For this review, take the finished solid that the model builds, in its own axes (mm). Face numbers are marked on the shaded views. A direction names the side the tool comes from. Round coordinates to 2 decimals unless told otherwise and drop trailing zeros. Order: outer loops, then holes, each group sorted by start corner. A loop starts at its lowest first (then second) coordinate and runs counter-clockwise, first axis right, second up. Notation, with made-up numbers: (42.5, 68) -> (85.5, 68) arc R26 cw to (85.5, 93) -> close; hole circle Ø10 at (42.25, 53). An arc over 180 degrees is marked (long way). Use a Markdown table: item, result. Add a question column.
1) Consider section A-A (z = -10.5). State the section outline as (x, y) points.
2) Draft analysis for pull direction X (two halves, no side actions). For the marked faces 6, 7 and 8, state which applies: pulls with the +X half, pulls with the -X half, needs draft (parallel to the pull), parting line crosses it, or undercut.
3) Consider section C-C (y = 12.5). State the section outline as (x, z) points, plus the area to 3 significant figures.
4) Clearance check with flat-ended pins moving along their axes: P1, Ø2, axis at y = 12.5, z = -7.5, coming from the -X side; P2, Ø6, axis at x = -32.5, z = 9.5, coming from the -Y side; P3, Ø2, axis at y = 2, z = -11, coming from the +X side; P4, Ø5, axis at x = -27, y = 9.5, coming from the +Z side. State where each tip first meets the part, or that it passes through.
5) Wall thickness on line 1 along X through (y, z) = (2.15, -10.5); line 2 along Y through (x, z) = (-28, -9); line 3 along Z through (x, y) = (-24, 12.5): over which ranges is each line inside the solid? List them lowest first. Write a range as [from, to].
6) Machinability: for the marked faces 1, 2, 3, 4 and 5, which of the approach directions +Z, -Z, +X, -X, +Y, -Y give a long, thin tool a straight path to every point of the face, cutting with its end or side? Answer none if there is none.
```python
from build123d import *

# Parameters (mm, degrees)
SKETCH1_W           = 15
SKETCH1_H           = 26
BOSS_EXTRUDE1_DEPTH = 3
CUT_EXTRUDE1_REACH  = 39.924
SKETCH2_R           = 1
SKETCH3_W           = 5
SKETCH3_H           = 10
BOSS_EXTRUDE2_DEPTH = 16
CUT_EXTRUDE2_REACH  = 29.477
SKETCH4_R           = 3
CUT_EXTRUDE3_REACH  = 43.052
SKETCH5_W           = 5
SKETCH5_H           = 8
SKETCH5_H_2         = 18
FILLET1_R           = 5
FILLET2_R           = 5
FILLET3_R           = 5
FILLET4_R           = 4
FILLET5_R           = 1


with BuildPart() as part:
    # Sketch1 → Boss-Extrude1 (new body)
    with BuildSketch(Plane(origin=(0, 0, 0), x_dir=(1, 0, 0), z_dir=(0, 1, 0))):
        with Locations((-28.000171023, 0)):
            Rectangle(SKETCH1_W, SKETCH1_H)
    extrude(amount=BOSS_EXTRUDE1_DEPTH)

    # Sketch2 → Cut-Extrude1 (cut, up to next)
    with BuildSketch(Plane(origin=(0, 3, 0), x_dir=(1, 0, 0), z_dir=(0, 1, 0)), mode=Mode.PRIVATE) as cut_extrude1_sk1:
        with Locations(Location((-32.666666667, -9.5, 0), (0, 0, 270))):
            Circle(SKETCH2_R)
    cut_extrude1_tool1 = extrude(cut_extrude1_sk1.sketch, amount=-CUT_EXTRUDE1_REACH, mode=Mode.PRIVATE) & part.part
    # Sketch2 → Cut-Extrude1 (cut, up to next)
    with BuildSketch(Plane(origin=(0, 3, 0), x_dir=(1, 0, 0), z_dir=(0, 1, 0)), mode=Mode.PRIVATE) as cut_extrude1_sk2:
        with Locations(Location((-28, 10.5, 0), (0, 0, 270))):
            Circle(SKETCH2_R)
    cut_extrude1_tool2 = extrude(cut_extrude1_sk2.sketch, amount=-CUT_EXTRUDE1_REACH, mode=Mode.PRIVATE) & part.part
    add(cut_extrude1_tool1.solids().sort_by_distance((-32.666667, 3, 9.5))[0], mode=Mode.SUBTRACT)
    add(cut_extrude1_tool2.solids().sort_by_distance((-28, 3, -10.5))[0], mode=Mode.SUBTRACT)

    # Sketch3 → Boss-Extrude2 (add)
    with BuildSketch(Plane(origin=(0, 3, 0), x_dir=(1, 0, 0), z_dir=(0, 1, 0))):
        with Locations((-23.000171023, 0)):
            Rectangle(SKETCH3_W, SKETCH3_H)
    extrude(amount=BOSS_EXTRUDE2_DEPTH)

    # Sketch4 → Cut-Extrude2 (cut, up to next)
    with BuildSketch(Plane(origin=(-20.500171023, 0, 0), x_dir=(0, 0, -1), z_dir=(1, 0, 0)), mode=Mode.PRIVATE) as cut_extrude2_sk1:
        with Locations((0, 14.5)):
            Circle(SKETCH4_R)
    cut_extrude2_tool1 = extrude(cut_extrude2_sk1.sketch, amount=-CUT_EXTRUDE2_REACH, mode=Mode.PRIVATE) & part.part
    add(cut_extrude2_tool1.solids().sort_by_distance((-20.500171, 14.5, 0))[0], mode=Mode.SUBTRACT)

    # Sketch5 → Cut-Extrude3 (cut, up to next)
    with BuildSketch(Plane(origin=(0, 3, 0), x_dir=(1, 0, 0), z_dir=(0, 1, 0)), mode=Mode.PRIVATE) as cut_extrude3_sk1:
        with Locations((-23.000171023, 9)):
            Rectangle(SKETCH5_W, SKETCH5_H)
    cut_extrude3_tool1 = extrude(cut_extrude3_sk1.sketch, amount=-CUT_EXTRUDE3_REACH, mode=Mode.PRIVATE) & part.part
    # Sketch5 → Cut-Extrude3 (cut, up to next)
    with BuildSketch(Plane(origin=(0, 3, 0), x_dir=(1, 0, 0), z_dir=(0, 1, 0)), mode=Mode.PRIVATE) as cut_extrude3_sk2:
        with Locations((-33.000171023, 4)):
            Rectangle(SKETCH5_W, SKETCH5_H_2)
    cut_extrude3_tool2 = extrude(cut_extrude3_sk2.sketch, amount=-CUT_EXTRUDE3_REACH, mode=Mode.PRIVATE) & part.part
    # Sketch5 → Cut-Extrude3 (cut, up to next)
    with BuildSketch(Plane(origin=(0, 3, 0), x_dir=(1, 0, 0), z_dir=(0, 1, 0)), mode=Mode.PRIVATE) as cut_extrude3_sk3:
        with Locations((-23.000171023, -9)):
            Rectangle(SKETCH5_W, SKETCH5_H)
    cut_extrude3_tool3 = extrude(cut_extrude3_sk3.sketch, amount=-CUT_EXTRUDE3_REACH, mode=Mode.PRIVATE) & part.part
    add(cut_extrude3_tool1.solids().sort_by_distance((-23.000171, 3, -9))[0], mode=Mode.SUBTRACT)
    add(cut_extrude3_tool2.solids().sort_by_distance((-33.000171, 3, -4))[0], mode=Mode.SUBTRACT)
    add(cut_extrude3_tool3.solids().sort_by_distance((-23.000171, 3, 9))[0], mode=Mode.SUBTRACT)

    # Fillet1
    fillet1_edges = [part.edges().sort_by_distance(p)[0] for p in [
        (-23.000171023, 19, -5),
        (-23.000171023, 19, 5),
    ]]
    fillet(fillet1_edges, radius=FILLET1_R - 0.0001)  # a hair under: the kernel refuses the full size

    # Fillet2
    fillet2_edges = [part.edges().sort_by_distance(p)[0] for p in [
        (-25.500171023, 3, 0),
    ]]
    fillet(fillet2_edges, radius=FILLET2_R - 0.0001)  # a hair under: the kernel refuses the full size

    # Fillet3
    fillet3_edges = [part.edges().sort_by_distance(p)[0] for p in [
        (-30.500171023, 1.5, 5),
        (-25.500171023, 1.5, -5),
        (-25.500171023, 1.5, 5),
    ]]
    fillet(fillet3_edges, radius=FILLET3_R - 0.0001)  # a hair under: the kernel refuses the full size

    # Fillet4
    fillet4_edges = [part.edges().sort_by_distance(p)[0] for p in [
        (-35.500171023, 1.5, 5),
        (-35.500171023, 1.5, 13),
        (-25.500171023, 1.5, 13),
    ]]
    fillet(fillet4_edges, radius=FILLET4_R)

    # Fillet5
    fillet5_edges = [part.edges().sort_by_distance(p)[0] for p in [
        (-30.500171023, 1.5, -13),
        (-25.500171023, 1.5, -13),
    ]]
    fillet(fillet5_edges, radius=FILLET5_R)


solid = part.part
```
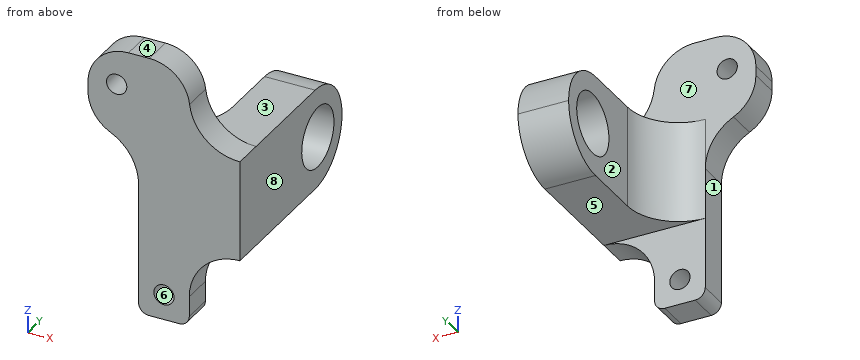
Results list:
| question | item | result |
|---|---|---|
| 1 | outline | (-30.5, 0) -> (-29, 0) -> (-29, 3) -> (-30.5, 3) -> close; (-27, 0) -> (-25.5, 0) -> (-25.5, 3) -> (-27, 3) -> close |
| 2 | face 6 | undercut |
| 2 | face 7 | needs draft |
| 2 | face 8 | pulls with the +X half |
| 3 | outline | (-25.5, -5) -> (-20.5, -5) -> (-20.5, -2.24) -> (-25.5, -2.24) -> close; (-25.5, 2.24) -> (-20.5, 2.24) -> (-20.5, 5) -> (-25.5, 5) -> close |
| 3 | area | 27.6 mm2 |
| 4 | P1 | through |
| 4 | P2 | y = 0 |
| 4 | P3 | x = -25.5 |
| 4 | P4 | z = 5 |
| 5 | line 1 | [-30.5, -29], [-27, -25.5] |
| 5 | line 2 | [0, 3] |
| 5 | line 3 | [-5, -2.24], [2.24, 5] |
| 6 | face 1 | -Z, -X, +Y, -Y |
| 6 | face 2 | +Z, -Z, -X, +Y |
| 6 | face 3 | +Z, +X, -X, +Y |
| 6 | face 4 | +Z, +X, -X, +Y, -Y |
| 6 | face 5 | -Z, +X, -X, +Y |
